Could you check a few things on this model? Use its own coordinates, in mm. A direction names the side the tool comes from. Round coordinates to 2 decimals unless told otherwise and drop trailing zeros. Write each loop counter-clockwise with the first axis right and the second up, starting at its lowest first coordinate (ties: lowest second). Pieces come first, ordered by that corner, then holes. Notation, with made-up numbers: (74.25, 5) -> (104.25, 5) arc R16 cw to (104.25, 18) -> close; hole circle Ø10 at (54, 13). An arc over 180 degrees is marked (long way). Answer in a Markdown table with one row per item.
from build123d import *

# Parameters (mm, degrees)
SKETCH1_R                = 4.5
BOSS_EXTRUDE1_DEPTH      = 6
BOSS_EXTRUDE2_DEPTH      = 1.75
BOSS_EXTRUDE2_DEPTH_BACK = 1.5
FILLET1_R                = 1


with BuildPart() as part:
    # Sketch1 → Boss-Extrude1 (new body)
    with BuildSketch(Plane.XY):
        with Locations((5.549376682, 2)):
            Circle(SKETCH1_R)
        Polygon((4.394676144, 0), (6.704077221, 0), (7.858777759, 2), (6.704077221, 4), (4.394676144, 4), (3.239975606, 2), align=None, mode=Mode.SUBTRACT)
    extrude(amount=BOSS_EXTRUDE1_DEPTH)

    # Sketch2 → Boss-Extrude2 (add, two sides)
    with BuildSketch(Plane(origin=(0, 2, 0), x_dir=(1, 0, 0), z_dir=(0, 1, 0))) as boss_extrude2_sk:
        Polygon((3.239975606, 0), (1.049376682, 0), (-1.950623318, 0), (-1.950623318, -6), (1.049376682, -6), (3.239975606, -6), align=None)
    extrude(amount=BOSS_EXTRUDE2_DEPTH)
    extrude(boss_extrude2_sk.sketch, amount=-BOSS_EXTRUDE2_DEPTH_BACK)

    # Fillet1
    fillet1_edges = [part.edges().sort_by_distance(p)[0] for p in [
        (-1.950623318, 3.75, 3),
        (-1.950623318, 0.5, 3),
    ]]
    fillet(fillet1_edges, radius=FILLET1_R)


solid = part.part
1) Please list where these lines run through material, in increasing order: line 1 (Y direction, x = 1, z = 0.5); line 2 (X direction, y = 1, z = 0.95); line 3 (Y direction, x = 4.5, z = 0.8).
Findings:
| item | result |
|---|---|
| line 1 | y = 0.5 to 3.75 |
| line 2 | x = -1.82 to 3.82, 7.28 to 9.94 |
| line 3 | y = -2.38 to 0, 4 to 6.38 |
2) For faces 1 (the face through (6, 0, 3)), 2 (the face through (0, 3.75, 3)), 3 (the face through (0, 0.5, 3)), which set-ups out of +Z, -Z, +X, -X, +Y, -Y let a thin tool reach every point of the face, with its end or its side?
Findings:
| item | result |
|---|---|
| face 1 | +Z, -Z |
| face 2 | +Z, -Z, -X, +Y |
| face 3 | +Z, -Z, -X, -Y |
3) Thinking about a two-plate mould opening in X: for faces 4 (the face through (-1.65, 3.465, 3.042)), 5 (the face through (3, 2, 6)), 6 (the face through (3.81, 1.01, 2.96)), which applies, +X half, -X half, draft (parallel to the pull), parting line (faces both ways), or undercut?
Findings:
| item | result |
|---|---|
| face 4 | -X half |
| face 5 | draft |
| face 6 | undercut |
4) For pin 1 (1.8 mm diameter, centred on x = -0.5, z = 2.5, fed in from -Y); pin 2 (3 mm diameter, centred on y = 3, z = 3.5, fed in from -X); pin 3 (1 mm diameter, centred on x = 0.5, z = 2.5, fed in from +Y); pin 4 (2.5 mm diameter, centred on x = 0, z = 2, fed in from +Y), each with a flat end and sliding along its axis, tell me the tip position at first contact or that it passes through.
Findings:
| item | result |
|---|---|
| pin 1 | stops at y = 0.5 |
| pin 2 | stops at x = -1.95 |
| pin 3 | stops at y = 3.75 |
| pin 4 | stops at y = 3.75 |
5) Imagine slicing it at B-B, the plane z = 4.15. Please give me the cut outline in (x, y).
Findings:
| item | result |
|---|---|
| outline | (-1.95, 1.5) arc R1 ccw to (-0.95, 0.5) -> (1.31, 0.5) arc R4.5 ccw (long way) to (1.4, 3.75) -> (-0.95, 3.75) arc R1 ccw to (-1.95, 2.75) -> close; hole (3.24, 2) -> (4.39, 0) -> (6.7, 0) -> (7.86, 2) -> (6.7, 4) -> (4.39, 4) -> close |
6) Imagine slicing it at D-D, the plane x = 2. Please give me the cut outline in (y, z), plus the area to 3 significant figures.
Findings:
| item | result |
|---|---|
| outline | (-0.77, 0) -> (4.77, 0) -> (4.77, 6) -> (-0.77, 6) -> close |
| area | 33.2 mm^2 |
7) Imagine slicing it at C-C, the plane x = 3.5. Please give me the cut outline in (y, z).
Findings:
| item | result |
|---|---|
| outline | (-2.01, 0) -> (1.55, 0) -> (1.55, 6) -> (-2.01, 6) -> close; (2.45, 0) -> (6.01, 0) -> (6.01, 6) -> (2.45, 6) -> close |
8) Imagine slicing it at A-A, the plane y = 1. Please give me the cut outline in (x, z).
Findings:
| item | result |
|---|---|
| outline | (-1.82, 0) -> (3.82, 0) -> (3.82, 6) -> (-1.82, 6) -> close; (7.28, 0) -> (9.94, 0) -> (9.94, 6) -> (7.28, 6) -> close |
